```python
from build123d import *

# Parameters (mm, degrees)
EXTRUDE015_DEPTH = 25
SKETCH011_R      = 4.125
EXTRUDE013_DEPTH = 4
SKETCH010_W      = 4
SKETCH010_H      = 84
SKETCH010_H_2    = 16
EXTRUDE012_DEPTH = 22


with BuildPart() as extrude015:
    # Sketch013 → Extrude015 (new body, symmetric)
    with BuildSketch(Plane.YZ):
        Polygon((-24, 0), (-22, 1.154701), (-20, 0), align=None)
    extrude(amount=EXTRUDE015_DEPTH, both=True)


with BuildPart() as extrude015_1:
    # Extrude015 placement: moved
    add(extrude015.part.moved(Location((0, 44, 0))))


with BuildPart() as cut001:
    # Sketch011 → Extrude013 (new body)
    with BuildSketch(Plane.XZ):
        Polygon((24, 0), (20, 0), (-20, 0), (-24, 0), (-24, 16), (-26, 17.154701), (-28, 16), (-69, 16), (-71, 17.154701), (-73, 16), (-73, 36.656854), (-25.656854, 84), (-20, 84), (20, 84), (24, 84), align=None)
        with Locations((-22, 20.125)):
            Circle(SKETCH011_R, mode=Mode.SUBTRACT)
    extrude(amount=EXTRUDE013_DEPTH)


with BuildPart() as cut001_1:
    # Extrude013 placement: moved
    add(cut001.part.moved(Location((0, 24, 0))))

    # Cut001: cut Extrude015
    add(extrude015_1.part, mode=Mode.SUBTRACT)


with BuildPart() as reject_path:
    # Sketch010 → Extrude012 (new body, symmetric)
    with BuildSketch(Plane.XZ):
        with Locations((22, 42)):
            Rectangle(SKETCH010_W, SKETCH010_H)
        with Locations((-22, 8)):
            Rectangle(SKETCH010_W, SKETCH010_H_2)
        Polygon((-20, 84), (-25.656854, 84), (-73, 36.656854), (-73, 16), (-71, 17.154701), (-69, 16), (-69, 35), (-24, 80), (-20, 80), align=None)
    extrude(amount=EXTRUDE012_DEPTH, both=True)


with BuildPart() as reject_path_1:
    # Extrude012 placement: moved
    add(reject_path.part.moved(Location((0, -2, 0))))

    # Fusion004: union Cut001
    add(cut001_1.part)


solid = reject_path_1.part
```
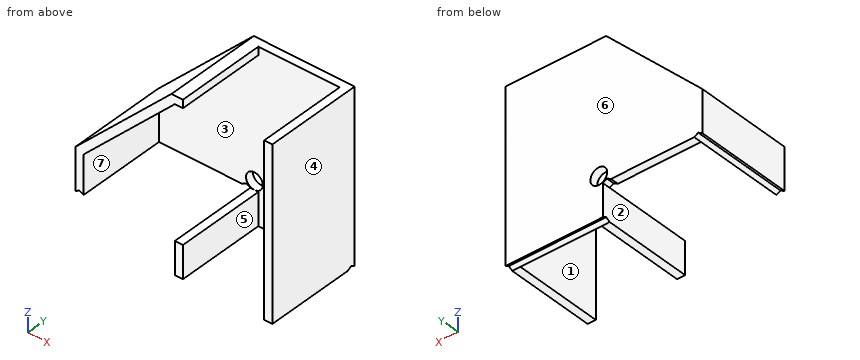
Build history of the part. All positions in model axes, mm. Face numbers are marked on the shaded views. A direction names the side the tool comes from. Round coordinates to 2 decimals unless told otherwise and drop trailing zeros. Order: outer loops, then holes, each group sorted by start corner. A loop starts at its lowest first (then second) coordinate and runs counter-clockwise, first axis right, second up. Notation, with made-up numbers: (59.25, 89.5) -> (72.25, 89.5) arc R12 cw to (72.25, 104.5) -> close; hole circle Ø6 at (13.25, 69). An arc over 180 degrees is marked (long way). Answer in a Markdown table with one row per item.
1) Band-saw the part on D-D on z = 55.5. Give the cut face in (x, y).
Values:
| item | result |
|---|---|
| outline | (-54.16, -24) -> (-48.5, -24) -> (-48.5, 20) -> (20, 20) -> (20, -24) -> (24, -24) -> (24, 24) -> (-54.16, 24) -> close |
2) Mould opens along X. For the marked faces 1, 2, 3 and 4 say: released by +X, released by -X, zero draft, split by the parting line, or undercut.
Values:
| item | result |
|---|---|
| face 1 | undercut |
| face 2 | released by -X |
| face 3 | undercut |
| face 4 | released by +X |
3) Pin check, flat tips, straight feed: P1, Ø1, axis at x = -53, y = -0.5, coming from the -Z side; P2, Ø6, axis at x = -17.5, z = 43, coming from the -Y side; P3, Ø1.5, axis at x = -35.5, y = 14.5, coming from the -Z side. Stop position of each tip, or through.
Values:
| item | result |
|---|---|
| P1 | z = 50.5 |
| P2 | y = 20 |
| P3 | z = 67.75 |
4) Wall check: L1, parallel to X at y = 12, z = 34.5; L2, parallel to X at y = 14, z = 13; L3, parallel to Y at x = 6, z = 25. Give the ranges that are in metal, low to high.
Values:
| item | result |
|---|---|
| L1 | -73 to -69, 20 to 24 |
| L2 | -24 to -20, 20 to 24 |
| L3 | 20 to 24 |
5) Which spindle directions (+Z, -Z, +X, -X, +Y, -Y) get a long thin tool onto all of the face, cutting with end or side? Do the marked faces 5, 6 and 7. Say none if no direction does.
Values:
| item | result |
|---|---|
| face 5 | +Z, -Z, -Y |
| face 6 | +Z, -Z, +X, -X, +Y |
| face 7 | -Z, -Y |
6) Band-saw the part on A-A on y = -10. Give the cut face in (x, z), and give its area (3 significant figures).
Values:
| item | result |
|---|---|
| outline | (-73, 16) -> (-71, 17.15) -> (-69, 16) -> (-69, 35) -> (-24, 80) -> (-20, 80) -> (-20, 84) -> (-25.66, 84) -> (-73, 36.66) -> close; (-24, 0) -> (-20, 0) -> (-20, 16) -> (-24, 16) -> close; (20, 0) -> (24, 0) -> (24, 84) -> (20, 84) -> close |
| area | 758 mm2 |
7) Band-saw the part on C-C on x = -8. Give the cut face in (y, z), and give its area (3 significant figures).
Values:
| item | result |
|---|---|
| outline | (20, 0) -> (22, 1.15) -> (24, 0) -> (24, 84) -> (20, 84) -> close |
| area | 334 mm2 |
8) Band-saw the part on B-B on z = 23. Give the cut face in (x, y).
Values:
| item | result |
|---|---|
| outline | (-73, -24) -> (-69, -24) -> (-69, 20) -> (-24.96, 20) -> (-24.96, 24) -> (-73, 24) -> close; (-19.04, 20) -> (20, 20) -> (20, -24) -> (24, -24) -> (24, 24) -> (-19.04, 24) -> close |
